Read the model definition and answer for the solid it produces. Units are mm, in the model's axes. Face numbers are marked on the shaded views. A direction names the side the tool comes from. Give positions to 0.01 mm unless a question says otherwise; leave off trailing zeros. Write each loop counter-clockwise with the first axis right and the second up, starting at its lowest first coordinate (ties: lowest second). Pieces come first, ordered by that corner, then holes. Notation, with made-up numbers: (-9, 5.25) - (-1, 5.25) arc R24 ccw to (-1, 39.25) - close; hole circle Ø4 at (83.5, -19). An arc over 180 degrees is marked (long way). Answer as CSV lines item,"result".
```python
from build123d import *

# Parameters (mm, degrees)
F0_R      = 2.5
F0_R_2    = 1.5
F1_DEPTH  = 6.5
F2_W      = 9
F2_H      = 9
F3_DEPTH  = 10
F4_R      = 2.5
F5_R      = 1
F3_FACE_R = 1.5
F6_DEPTH  = 10
F7_R      = 3
F8_DEPTH  = 4


with BuildPart() as f1:
    # F0 (on Top) → F1 (new body)
    with BuildSketch(Plane.XY):
        Circle(F0_R)
        Circle(F0_R_2, mode=Mode.SUBTRACT)
    extrude(amount=F1_DEPTH)

    # F2 (on face) → F3 (join)
    with BuildSketch(Plane.XY.offset(6.5)):
        Rectangle(F2_W, F2_H)
    extrude(amount=F3_DEPTH)

    # F4
    f4_edges = [f1.edges().sort_by_distance(p)[0] for p in [
        (-4.5, -4.5, 11.5),
        (4.5, -4.5, 11.5),
        (4.5, 4.5, 11.5),
        (-4.5, 4.5, 11.5),
    ]]
    fillet(f4_edges, radius=F4_R)

    # F5
    f5_edges = [f1.edges().sort_by_distance(p)[0] for p in [
        (-4.5, 0, 6.5),
        (-4.5, 0, 16.5),
    ]]
    fillet(f5_edges, radius=F5_R)

    # F3_face (on face) → F6 (cut)
    with BuildSketch(Plane(origin=(0, 0, 6.5), x_dir=(1, 0, 0), z_dir=(0, 0, -1))):
        Circle(F3_FACE_R)
    extrude(amount=-F6_DEPTH, mode=Mode.SUBTRACT)

    # F7 (on face) → F8 (cut)
    with BuildSketch(Plane.XY.offset(16.5)):
        Circle(F7_R)
    extrude(amount=-F8_DEPTH, mode=Mode.SUBTRACT)


solid = f1.part
```
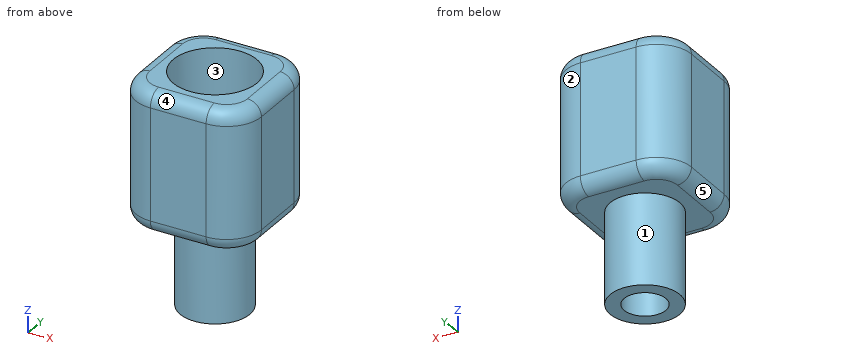
(1) The mould has two halves that part along Y. Classify the marked faces 3, 4 and 5: +Y half, -Y half, draft (parallel to the pull), parting line (faces both ways), or undercut.
Worked out:
face 3,"undercut"
face 4,"-Y half"
face 5,"draft"
(2) Each of these flat-tipped pins is pushed along its axis until it touches: P1, Ø5, axis at x = 1.5, y = 2, coming from the -Z side; P2, Ø5, axis at x = 0.5, z = 4.5, coming from the +Y side. Where does it stop, or does it pass through?
Worked out:
P1,"stops at z = 0"
P2,"stops at y = 4.37"
(3) A cutting plane is placed at B-B (z = 14.25). Write down the section's boundary in (x, y).
Worked out:
outline,"(-4.5, -2) arc R2.5 ccw to (-2, -4.5) - (2, -4.5) arc R2.5 ccw to (4.5, -2) - (4.5, 2) arc R2.5 ccw to (2, 4.5) - (-2, 4.5) arc R2.5 ccw to (-4.5, 2) - close; hole circle Ø6 at (0, 0)"
(4) A cutting plane is placed at A-A (y = 0). Write down the section's boundary in (x, z).
Worked out:
outline,"(-4.5, 7.5) arc R1 ccw to (-3.5, 6.5) - (-2.5, 6.5) - (-2.5, 0) - (-1.5, 0) - (-1.5, 12.5) - (-3, 12.5) - (-3, 16.5) - (-3.5, 16.5) arc R1 ccw to (-4.5, 15.5) - close; (1.5, 0) - (2.5, 0) - (2.5, 6.5) - (3.5, 6.5) arc R1 ccw to (4.5, 7.5) - (4.5, 15.5) arc R1 ccw to (3.5, 16.5) - (3, 16.5) - (3, 12.5) - (1.5, 12.5) - close"
(5) A cutting plane is placed at D-D (z = 12). Write down the section's boundary in (x, y).
Worked out:
outline,"(-4.5, -2) arc R2.5 ccw to (-2, -4.5) - (2, -4.5) arc R2.5 ccw to (4.5, -2) - (4.5, 2) arc R2.5 ccw to (2, 4.5) - (-2, 4.5) arc R2.5 ccw to (-4.5, 2) - close; hole circle Ø3 at (0, 0)"
(6) Find the intervals of material crossed by L1, parallel to Y at x = 0, z = 14.15; L2, parallel to Y at x = 0, z = 3; L3, parallel to Z at x = 3, y = -0.75, in increasing order.
Worked out:
L1,"y = -4.5 to -3, 3 to 4.5"
L2,"y = -2.5 to -1.5, 1.5 to 2.5"
L3,"z = 6.5 to 16.5"
(7) For the marked faces 1 and 2, determine the directions among +Z, -Z, +X, -X, +Y, -Y from which every point of the face is accessible in a straight line to the end or side of a thin tool.
Worked out:
face 1,"-Z"
face 2,"+Z, -Z, +X, +Y"
